Answer from the drawing. Dimensions are ordinates in mm from the lowest x, y and z of the part. A direction names the side the tool comes from. Round coordinates to 2 decimals unless told otherwise and drop trailing zeros. Write each loop counter-clockwise with the first axis right and the second up, starting at its lowest first coordinate (ties: lowest second). Pieces come first, ordered by that corner, then holes.
1. Find section A-A (x = 12.5). Write down the section's boundary in (y, z), and give its area (3 significant figures).
2. Straight lines are drawn through the part: probe 1 along Z at (x, y) = (97.5, 1.5); probe 2 along Z at (x, y) = (12.5, 11); probe 3 along Y at (x, z) = (99, 3). For each, find the intervals that lie inside material, in ascending order.
3. Flat-ended cylindrical pins translate along their axes: pin 1 Ø12 at (x, z) = (13.5, 19) entering from -Y; pin 2 Ø1 at (y, z) = (5, 9) entering from +X; pin 3 Ø1 at (x, y) = (55.5, 6) entering from +Z. Find the tip coordinate at first contact, or state that the pin passes through.
4. A tool of negligible diameter and unlimited length cuts with its end or side. For the marked faces 1, 2 and 3, from which of +Z, -Z, +X, -X, +Y, -Y can it reach the whole face along a straight path? Write none if from no direction.
5. Find section D-D (x = 97.5). Write down the section's boundary in (y, z), and give its area (3 significant figures).
6. Find section C-C (y = 4). Write down the section's boundary in (x, z) (1 decimal), and give its area (3 significant figures).
7. Find section B-B (z = 13.5). Write down the section's boundary in (x, y).
8. Determine the mould class of the marked faces 4, 5, 6 and 7 for opening direction Z: pulls with the +Z half, pulls with the -Z half, needs draft (parallel to the pull), parting line crosses it, or undercut.
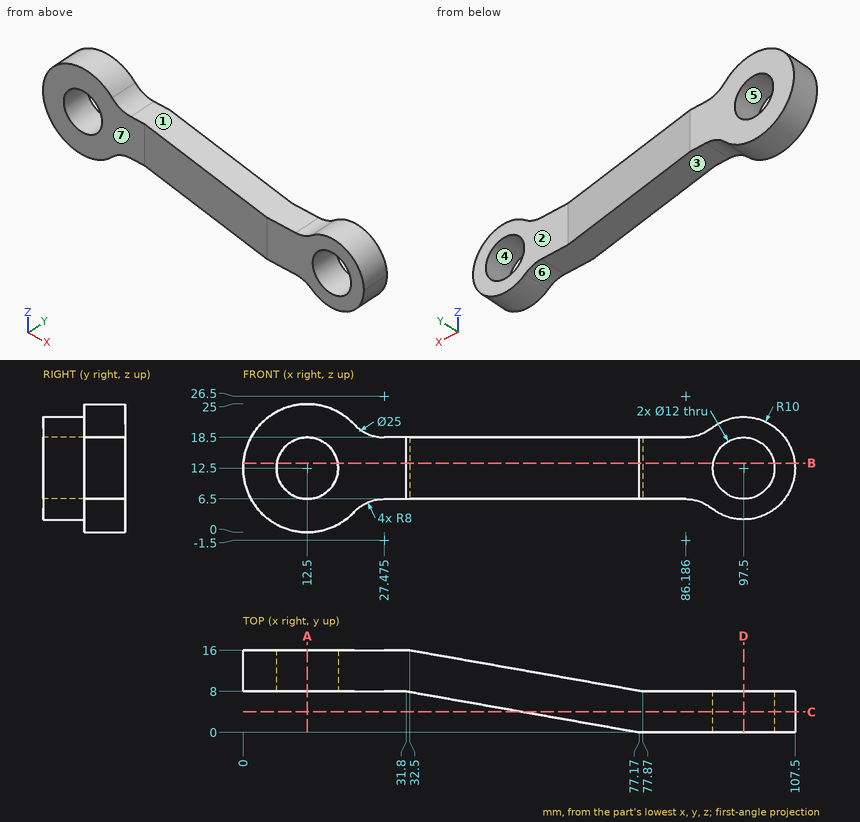
Worked answers:
1. outline: (8, 0) - (16, 0) - (16, 6.5) - (8, 6.5) - close; (8, 18.5) - (16, 18.5) - (16, 25) - (8, 25) - close
1. area: 104 mm2
2. probe 1: z = 2.5 to 6.5, 18.5 to 22.5
2. probe 2: z = 0 to 6.5, 18.5 to 25
2. probe 3: y = 0 to 8
3. pin 1: stops at y = 8
3. pin 2: stops at x = 107.04
3. pin 3: stops at z = 18.5
4. face 1: +Z, +Y, -Y
4. face 2: +Z, -Z, +X, +Y
4. face 3: -Z, +Y, -Y
5. outline: (0, 2.5) - (8, 2.5) - (8, 6.5) - (0, 6.5) - close; (0, 18.5) - (8, 18.5) - (8, 22.5) - (0, 22.5) - close
5. area: 64.0 mm2
6. outline: (54.5, 6.5) - (86.2, 6.5) arc R8 cw to (91.2, 4.7) arc R10 ccw (long way) to (91.2, 20.3) arc R8 cw to (86.2, 18.5) - (54.5, 18.5) - close; hole circle Ø12 at (97.5, 12.5)
6. area: 607 mm2
7. outline: (0.04, 8) - (6.58, 8) - (6.58, 16) - (0.04, 16) - close; (18.42, 8) - (31.8, 8) - (77.17, 0) - (91.58, 0) - (91.58, 8) - (77.87, 8) - (32.5, 16) - (18.42, 16) - close; (103.42, 0) - (107.45, 0) - (107.45, 8) - (103.42, 8) - close
8. face 4: undercut
8. face 5: undercut
8. face 6: pulls with the -Z half
8. face 7: needs draft
